from build123d import *

# Parameters (mm, degrees)
SKETCH1_W                  = 35
SKETCH1_H                  = 35
SKETCH1_R                  = 1.5
SKETCH1_R_2                = 5
BOSS_EXTRUDE1_DEPTH        = 0.79375
CONVERT_SOLID2_START       = -0.79375
CONVERT_SOLID2_OUTLINE_W   = 35
CONVERT_SOLID2_OUTLINE_H   = 35
CONVERT_SOLID2_OUTLINE_R   = 1.5
CONVERT_SOLID2_OUTLINE_R_2 = 5
CONVERT_SOLID2_DEPTH       = 0.79375
EDGE_FLANGE1_DEPTH         = 35
EDGE_FLANGE2_DEPTH         = 35
SKETCH24_R                 = 12.4
CUT_EXTRUDE1_DEPTH         = 10
SKETCH29_W                 = 15
SKETCH29_H                 = 20
TAB1_DEPTH                 = 1.5875
SKETCH32_W                 = 15
SKETCH32_H                 = 20
TAB2_DEPTH                 = 1.5875
SKETCH35_R                 = 2.2225
CUT_EXTRUDE2_DEPTH         = 10


# Read off the part's stored shape, not the designer's step: Convert-Solid2
# Sheet-metal steps are written as plain solids
with BuildPart() as part:
    # Sketch1 → Boss-Extrude1 (new body)
    with BuildSketch(Plane.XY):
        Rectangle(SKETCH1_W, SKETCH1_H)
        with Locations((-8.5, 0)):
            Circle(SKETCH1_R, mode=Mode.SUBTRACT)
        with Locations((8.5, 0)):
            Circle(SKETCH1_R, mode=Mode.SUBTRACT)
        Circle(SKETCH1_R_2, mode=Mode.SUBTRACT)
    extrude(amount=BOSS_EXTRUDE1_DEPTH)

    # Convert-Solid2 outline → Convert-Solid2 (add)
    with BuildSketch(Plane.XY.offset(CONVERT_SOLID2_START)):
        Rectangle(CONVERT_SOLID2_OUTLINE_W, CONVERT_SOLID2_OUTLINE_H)
        with Locations((-8.5, 0)):
            Circle(CONVERT_SOLID2_OUTLINE_R, mode=Mode.SUBTRACT)
        Circle(CONVERT_SOLID2_OUTLINE_R_2, mode=Mode.SUBTRACT)
        with Locations((8.5, 0)):
            Circle(CONVERT_SOLID2_OUTLINE_R, mode=Mode.SUBTRACT)
    extrude(amount=CONVERT_SOLID2_DEPTH)

    # Edge-Flange1 section (across the edge) → Edge-Flange1 (add)
    with BuildSketch(Plane(origin=(17.5, -18.77, -0.79375), x_dir=(0, 1, 0), z_dir=(-1, 0, 0))):
        with BuildLine():
            Line((-1.5875, 1.27), (-1.5875, 35))
            Line((-1.5875, 35), (0, 35))
            Line((0, 35), (0, 1.27))
            ThreePointArc((0, 1.27), (0.371974388, 0.371974388), (1.27, 0))
            Line((1.27, 0), (1.27, -1.5875))
            ThreePointArc((1.27, -1.5875), (-0.750557627, -0.750557627), (-1.5875, 1.27))
        make_face()
    extrude(amount=EDGE_FLANGE1_DEPTH)

    # Edge-Flange2 section (across the edge) → Edge-Flange2 (add)
    with BuildSketch(Plane(origin=(17.5, -18.77, -36.79375), x_dir=(0, 0, 1), z_dir=(-1, 0, 0))):
        with BuildLine():
            Line((-1.5875, 1), (-1.5875, 36))
            Line((-1.5875, 36), (0, 36))
            Line((0, 36), (0, 1))
            ThreePointArc((0, 1), (0.292893219, 0.292893219), (1, 0))
            Line((1, 0), (1, -1.5875))
            ThreePointArc((1, -1.5875), (-0.829638796, -0.829638796), (-1.5875, 1))
        make_face()
    extrude(amount=EDGE_FLANGE2_DEPTH)

    # Sketch24 → Cut-Extrude1 (cut)
    with BuildSketch(Plane(origin=(0, 0, -38.38125), x_dir=(-1, 0, 0), z_dir=(0, 0, -1))):
        with Locations(Location((0, 0, 0), (0, 0, 90))):
            Circle(SKETCH24_R)
    extrude(amount=-CUT_EXTRUDE1_DEPTH, mode=Mode.SUBTRACT)

    # Sketch29 → Tab1 (add)
    with BuildSketch(Plane(origin=(0, -18.77, 0), x_dir=(1, 0, 0), z_dir=(0, 1, 0))):
        with Locations((25, 18.92875)):
            Rectangle(SKETCH29_W, SKETCH29_H)
    extrude(amount=-TAB1_DEPTH)

    # Sketch32 → Tab2 (add)
    with BuildSketch(Plane(origin=(0, -18.77, 0), x_dir=(1, 0, 0), z_dir=(0, 1, 0))):
        with Locations((-25, 18.92875)):
            Rectangle(SKETCH32_W, SKETCH32_H)
    extrude(amount=-TAB2_DEPTH)

    # Sketch35 → Cut-Extrude2 (cut)
    with BuildSketch(Plane(origin=(0, -18.77, 0), x_dir=(1, 0, 0), z_dir=(0, 1, 0))):
        with Locations(Location((22.5, 13.92875, 0), (0, 0, 270))):
            Circle(SKETCH35_R)
        with Locations(Location((27.5, 23.92875, 0), (0, 0, 270))):
            Circle(SKETCH35_R)
    cut_extrude2 = extrude(amount=-CUT_EXTRUDE2_DEPTH, mode=Mode.SUBTRACT)

    # Mirror1: Cut-Extrude2 across plane
    add(cut_extrude2.mirror(Plane(origin=(0, 0, 0), x_dir=(0, 0, 1), z_dir=(1, 0, 0))), mode=Mode.SUBTRACT)


solid = part.part
Could you check a few things on this model? Use its own coordinates, in mm. A direction names the side the tool comes from. Coordinates: 2 decimals unless noted, no trailing zeros. Order: outer loops, then holes, each group sorted by start corner. A loop starts at its lowest first (then second) coordinate and runs counter-clockwise, first axis right, second up. Notation, with made-up numbers: (62, -12) - (115, -12) arc R24 ccw to (115, -1) - close; hole circle Ø10 at (-30, 31). An arc over 180 degrees is marked (long way). Answer in a Markdown table with one row per item. Add a question column.
(1) On a 3-axis mill with a long thin cutter (end or side, diameter ignored), from which of +Z, -Z, +X, -X, +Y, -Y can I reach the whole of each face in a straight line? I mean faces 4 (the face through (-17.5, -4, 0)), 5 (the face through (0, 17.23, -38)), 6 (the face through (0, -18.77, -19)), 7 (the face through (17.5, -4, -37)). Say none if no direction works.
(2) If we section it at A-A, the plane x = -1: Please give me the cut outline in (y, z) (1 decimal).
(3) If we section it at B-B, the plane y = 10: Please give me the cut outline in (x, z).
(4) Will these pins go through, and if not, where does the flat tip stop? pin 1 (0.5 mm diameter, centred on x = 25, y = -19.5, fed in from +Z); pin 2 (17 mm diameter, centred on x = 3, z = -21, fed in from +Y); pin 3 (1.7 mm diameter, centred on x = 23, y = -19.5, fed in from -Z).
(5) If we section it at D-D, the plane z = -17: Please give me the cut outline in (x, y), then the cut area to 3 significant figures.
(6) I need wall thicknesses on L1, parallel to Z at x = -16, y = 7; L2, parallel to Y at x = -8, z = 0; L3, parallel to Y at x = -8.5, z = -0.5. Which ranges of each line are inside material? Lowest first, please.
(7) If we section it at C-C, the plane x = -22.5: Please give me the cut outline in (y, z), then the cut area to 3 significant figures.
(8) If we mould it in two halves opening along X, with no side actions, what happens to faces 1 (the face through (24, -19.55, -15.57)), 2 (the face through (25, -20, -28.929)), 3 (the face through (-32.5, -20, -19))? For each: released by +X, released by -X, zero draft, split by the parting line, or undercut.
Results are:
| question | item | result |
|---|---|---|
| 1 | face 4 | +Z, -X, +Y, -Y |
| 1 | face 5 | -Z, +X, -X, +Y |
| 1 | face 6 | +X, -X, +Y |
| 1 | face 7 | -Z, +X, +Y, -Y |
| 2 | outline | (-20.4, -35.8) arc R2.6 ccw to (-17.8, -38.4) - (-12.4, -38.4) - (-12.4, -36.8) - (-17.8, -36.8) arc R1 cw to (-18.8, -35.8) - (-18.8, -2.1) arc R1.3 cw to (-17.5, -0.8) - (-4.9, -0.8) - (-4.9, 0.8) - (-17.5, 0.8) arc R2.9 ccw to (-20.4, -2.1) - close; (4.9, -0.8) - (17.5, -0.8) - (17.5, 0.8) - (4.9, 0.8) - close; (12.4, -38.4) - (17.2, -38.4) - (17.2, -36.8) - (12.4, -36.8) - close |
| 3 | outline | (-17.5, -38.38) - (-7.33, -38.38) - (-7.33, -36.79) - (-17.5, -36.79) - close; (-17.5, -0.79) - (17.5, -0.79) - (17.5, 0.79) - (-17.5, 0.79) - close; (7.33, -38.38) - (17.5, -38.38) - (17.5, -36.79) - (7.33, -36.79) - close |
| 4 | pin 1 | stops at z = -8.93 |
| 4 | pin 2 | stops at y = -18.77 |
| 4 | pin 3 | stops at z = -28.93 |
| 5 | outline | (-32.5, -20.36) - (32.5, -20.36) - (32.5, -18.77) - (-32.5, -18.77) - close |
| 5 | area | 103 mm2 |
| 6 | L1 | z = -38.38 to -36.79, -0.79 to 0.79 |
| 6 | L2 | y = -19.48 to -1.41, 1.41 to 17.5 |
| 6 | L3 | y = -19.89 to -1.5, 1.5 to 17.5 |
| 7 | outline | (-20.36, -28.93) - (-18.77, -28.93) - (-18.77, -16.15) - (-20.36, -16.15) - close; (-20.36, -11.71) - (-18.77, -11.71) - (-18.77, -8.93) - (-20.36, -8.93) - close |
| 7 | area | 24.7 mm2 |
| 8 | face 1 | undercut |
| 8 | face 2 | zero draft |
| 8 | face 3 | released by -X |
